Model file for the job. Use its own axes, mm. Face numbers are marked on the shaded views. A direction names the side the tool comes from. Round coordinates to 2 decimals unless told otherwise and drop trailing zeros. Order: outer loops, then holes, each group sorted by start corner. A loop starts at its lowest first (then second) coordinate and runs counter-clockwise, first axis right, second up. Notation, with made-up numbers: (75.5, -34.5) -> (118.5, -34.5) arc R26 ccw to (118.5, 3.5) -> close; hole circle Ø6 at (-15.75, -9). An arc over 180 degrees is marked (long way). Use CSV: the item, a comma, the result in double quotes.
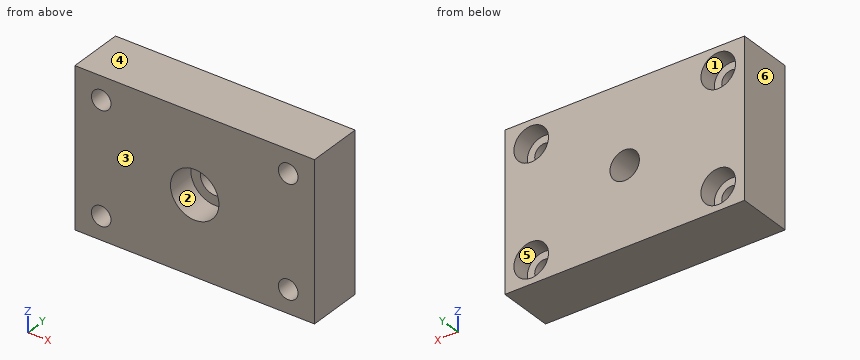
```python
from build123d import *

# Parameters (mm, degrees)
SKETCH1_W                                        = 55
SKETCH1_H                                        = 36
BOSS_EXTRUDE1_DEPTH                              = 12.7
CBORE_FOR_8_SOCKET_HEAD_CAP_SCREW1_D             = 4.4958
CBORE_FOR_8_SOCKET_HEAD_CAP_SCREW1_CBORE_D       = 7.9375
CBORE_FOR_8_SOCKET_HEAD_CAP_SCREW1_CBORE_DEPTH   = 4.1656
CBORE_FOR_1_4_SOCKET_HEAD_CAP_SCREW1_D           = 6.7564
CBORE_FOR_1_4_SOCKET_HEAD_CAP_SCREW1_CBORE_D     = 11.1125
CBORE_FOR_1_4_SOCKET_HEAD_CAP_SCREW1_CBORE_DEPTH = 6.35


with BuildPart() as part:
    # Sketch1 → Boss-Extrude1 (new body)
    with BuildSketch(Plane(origin=(0, 0, 0), x_dir=(1, 0, 0), z_dir=(0, 1, 0))):
        Rectangle(SKETCH1_W, SKETCH1_H)
    extrude(amount=BOSS_EXTRUDE1_DEPTH)

    # CBORE for #8 Socket Head Cap Screw1 (through all)
    with Locations(Plane(origin=(0, 12.7, 0), x_dir=(-1, 0, 0), z_dir=(0, 1, 0))):
        with Locations((21.463, -12.7), (21.463, 12.7), (-21.463, 12.7), (-21.463, -12.7)):
            CounterBoreHole(CBORE_FOR_8_SOCKET_HEAD_CAP_SCREW1_D / 2, CBORE_FOR_8_SOCKET_HEAD_CAP_SCREW1_CBORE_D / 2, CBORE_FOR_8_SOCKET_HEAD_CAP_SCREW1_CBORE_DEPTH)

    # CBORE for 1/4 Socket Head Cap Screw1 (through all)
    with Locations(Plane(origin=(0, 0, 0), x_dir=(-1, 0, 0), z_dir=(0, -1, 0))):
        with Locations((0, 0)):
            CounterBoreHole(CBORE_FOR_1_4_SOCKET_HEAD_CAP_SCREW1_D / 2, CBORE_FOR_1_4_SOCKET_HEAD_CAP_SCREW1_CBORE_D / 2, CBORE_FOR_1_4_SOCKET_HEAD_CAP_SCREW1_CBORE_DEPTH)


solid = part.part
```
Q1. Which spindle directions (+Z, -Z, +X, -X, +Y, -Y) get a long thin tool onto all of the face, cutting with end or side? Do the marked faces 5 and 6. Say none if no direction does.
From the geometry:
face 5,"+Y"
face 6,"+Z, -Z, -X, +Y, -Y"
Q2. Cut at C-C (y = 7). Give the cut face in (x, z), plus the area to 3 significant figures.
From the geometry:
outline,"(-27.5, -18) -> (27.5, -18) -> (27.5, 18) -> (-27.5, 18) -> close; hole circle Ø4.5 at (-21.46, -12.7); hole circle Ø4.5 at (-21.46, 12.7); hole circle Ø6.76 at (0, 0); hole circle Ø4.5 at (21.46, -12.7); hole circle Ø4.5 at (21.46, 12.7)"
area,"1,880 mm²"
Q3. Cut at B-B (x = 0). Give the cut face in (y, z), plus the area to 3 significant figures.
From the geometry:
outline,"(0, -18) -> (12.7, -18) -> (12.7, -3.38) -> (6.35, -3.38) -> (6.35, -5.56) -> (0, -5.56) -> close; (0, 5.56) -> (6.35, 5.56) -> (6.35, 3.38) -> (12.7, 3.38) -> (12.7, 18) -> (0, 18) -> close"
area,"344 mm²"
Q4. Pin check, flat tip, straight feed: pin 1 (6.5 mm diameter, centred on x = 21.463, z = 12.7, fed in from +Y). Stop position of the tip, or through.
From the geometry:
pin 1,"stops at y = 8.53"
Q5. Cut at A-A (z = -12.7). Give the cut face in (x, y), plus the area to 3 significant figures.
From the geometry:
outline,"(-27.5, 0) -> (-23.71, 0) -> (-23.71, 8.53) -> (-25.43, 8.53) -> (-25.43, 12.7) -> (-27.5, 12.7) -> close; (-19.22, 0) -> (19.22, 0) -> (19.22, 8.53) -> (17.49, 8.53) -> (17.49, 12.7) -> (-17.49, 12.7) -> (-17.49, 8.53) -> (-19.22, 8.53) -> close; (23.71, 0) -> (27.5, 0) -> (27.5, 12.7) -> (25.43, 12.7) -> (25.43, 8.53) -> (23.71, 8.53) -> close"
area,"556 mm²"
Q6. Probe line 1 along X through (y, z) = (12, 13); line 2 along X through (y, z) = (4, 12.5); line 3 along Z through (x, y) = (23, 6.5). List the from-to ranges inside material, lowest first.
From the geometry:
line 1,"x = -27.5 to -25.42, -17.51 to 17.51, 25.42 to 27.5"
line 2,"x = -27.5 to -23.7, -19.22 to 19.22, 23.7 to 27.5"
line 3,"z = -18 to -14.34, -11.06 to 11.06, 14.34 to 18"
Q7. Mould opens along Z. For the marked faces 1, 2, 3 and 4 say: +Z half, -Z half, draft (parallel to the pull), parting line (faces both ways), or undercut.
From the geometry:
face 1,"undercut"
face 2,"undercut"
face 3,"draft"
face 4,"+Z half"
Q8. Cut at D-D (z = 0). Give the cut face in (x, y).
From the geometry:
outline,"(-27.5, 0) -> (-5.56, 0) -> (-5.56, 6.35) -> (-3.38, 6.35) -> (-3.38, 12.7) -> (-27.5, 12.7) -> close; (3.38, 6.35) -> (5.56, 6.35) -> (5.56, 0) -> (27.5, 0) -> (27.5, 12.7) -> (3.38, 12.7) -> close"
